```python
from build123d import *

# Parameters (mm, degrees)
BOSS_EXTRUDE1_DEPTH = 50.8
SKETCH2_W           = 28.5
SKETCH2_H           = 19.05
SKETCH2_H_2         = 62.95
SKETCH2_W_2         = 13.15
SKETCH2_H_3         = 42
CUT_EXTRUDE2_DEPTH  = 150
SKETCH8_R           = 9.625
CUT_EXTRUDE8_DEPTH  = 90.793902911
SKETCH11_R          = 9.625
SKETCH11_W          = 8.25
SKETCH11_H          = 8.25
BOSS_EXTRUDE4_DEPTH = 5.15
FILLET1_R           = 6
CUT_EXTRUDE10_START = -5.15
SKETCH14_R          = 1.5875
CUT_EXTRUDE10_DEPTH = 5.15
CUT_EXTRUDE16_REACH = 91.794
SKETCH21_R          = 3


with BuildPart() as part:
    # Sketch1 → Boss-Extrude1 (new body)
    with BuildSketch(Plane(origin=(0, 0, 0), x_dir=(0, 0, -1), z_dir=(1, 0, 0))):
        with BuildLine():
            Line((-52.5, 19.05), (52.5, 19.05))
            ThreePointArc((52.5, 19.05), (71.55, 0), (52.5, -19.05))
            Line((52.5, -19.05), (-52.5, -19.05))
            ThreePointArc((-52.5, -19.05), (-71.55, 0), (-52.5, 19.05))
        make_face()
    extrude(amount=BOSS_EXTRUDE1_DEPTH)

    # Sketch2 → Cut-Extrude2 (cut)
    with BuildSketch(Plane(origin=(0, 19.05, 0), x_dir=(1, 0, 0), z_dir=(0, 1, 0))):
        with Locations((25.4, 62.025)):
            Rectangle(SKETCH2_W, SKETCH2_H)
        with Locations((25.4, 21.025)):
            Rectangle(SKETCH2_W, SKETCH2_H_2)
        with Locations((44.225, -50.55)):
            Rectangle(SKETCH2_W_2, SKETCH2_H_3)
        with Locations((6.575, -50.55)):
            Rectangle(SKETCH2_W_2, SKETCH2_H_3)
    extrude(amount=-CUT_EXTRUDE2_DEPTH, mode=Mode.SUBTRACT)

    # Sketch8 → Cut-Extrude8 (cut, through all)
    with BuildSketch(Plane(origin=(50.8, 0, 0), x_dir=(0, 0, -1), z_dir=(1, 0, 0))):
        with Locations((-52.5, 0)):
            Circle(SKETCH8_R)
        with Locations((52.5, 0)):
            Circle(SKETCH8_R)
    extrude(amount=-CUT_EXTRUDE8_DEPTH, mode=Mode.SUBTRACT)

    # Sketch11 → Boss-Extrude4 (add)
    with BuildSketch(Plane(origin=(50.8, 0, 0), x_dir=(0, 0, -1), z_dir=(1, 0, 0))):
        with Locations((52.5, 0)):
            Circle(SKETCH11_R)
        with Locations((52.5, 0)):
            Rectangle(SKETCH11_W, SKETCH11_H, mode=Mode.SUBTRACT)
    extrude(amount=-BOSS_EXTRUDE4_DEPTH)

    # Fillet1
    fillet1_edges = [part.edges().sort_by_distance(p)[0] for p in [
        (50.8, 0, 29.55),
        (0, 0, 29.55),
    ]]
    fillet(fillet1_edges, radius=FILLET1_R)

    # Sketch14 → Cut-Extrude10 (cut)
    with BuildSketch(Plane(origin=(50.8, 0, 0), x_dir=(0, 0, -1), z_dir=(1, 0, 0)).offset(CUT_EXTRUDE10_START)):
        with Locations((49.497532015, 3.002467985)):
            Circle(SKETCH14_R)
        with Locations((55.502467985, 3.002467985)):
            Circle(SKETCH14_R)
        with Locations((55.502467985, -3.002467985)):
            Circle(SKETCH14_R)
        with Locations((49.497532015, -3.002467985)):
            Circle(SKETCH14_R)
    extrude(amount=CUT_EXTRUDE10_DEPTH, mode=Mode.SUBTRACT)

    # Sketch21 → Cut-Extrude16 (cut, up to next)
    with BuildSketch(Plane.ZY, mode=Mode.PRIVATE) as cut_extrude16_sk1:
        with Locations((-12.5, 13)):
            Circle(SKETCH21_R)
    cut_extrude16_tool1 = extrude(cut_extrude16_sk1.sketch, amount=-CUT_EXTRUDE16_REACH, mode=Mode.PRIVATE) & part.part
    # Sketch21 → Cut-Extrude16 (cut, up to next)
    with BuildSketch(Plane.ZY, mode=Mode.PRIVATE) as cut_extrude16_sk2:
        with Locations((-12.5, -13)):
            Circle(SKETCH21_R)
    cut_extrude16_tool2 = extrude(cut_extrude16_sk2.sketch, amount=-CUT_EXTRUDE16_REACH, mode=Mode.PRIVATE) & part.part
    add(cut_extrude16_tool1.solids().sort_by_distance((0, 13, -12.5))[0], mode=Mode.SUBTRACT)
    add(cut_extrude16_tool2.solids().sort_by_distance((0, -13, -12.5))[0], mode=Mode.SUBTRACT)


solid = part.part
```
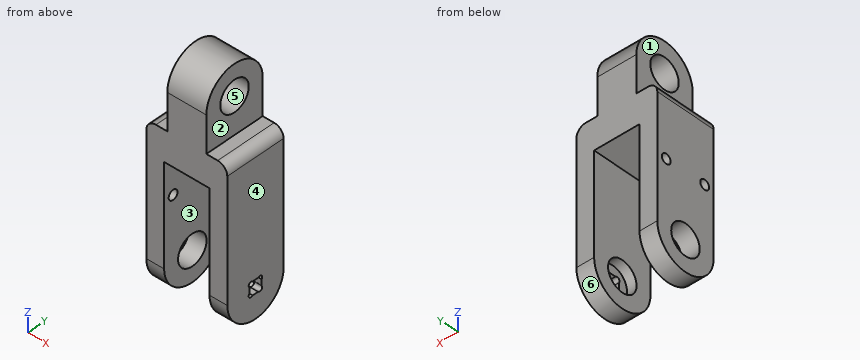
Geometry: final body of the model. Coordinates: model frame, mm. Face numbers are marked on the shaded views. A direction names the side the tool comes from. Give positions to 0.01 mm unless a question says otherwise; leave off trailing zeros. Loops run counter-clockwise (first coordinate to the right, second up) from the corner with the lowest first, then second, coordinate; pieces in that order, holes last. Notation, with made-up numbers: (-23, 57) -> (-10, 57) arc R11 cw to (-10, 68) -> close; hole circle Ø9 at (63, 30). An arc over 180 degrees is marked (long way). Use one line per item in the form item = value.
Item 1: Section query B-B on z = -31. Output: boundary loops of the cut face in (x, y), and give its area (3 significant figures).
A:
outline = (0, -19.05) -> (11.15, -19.05) -> (11.15, 19.05) -> (0, 19.05) -> close; (39.65, -19.05) -> (50.8, -19.05) -> (50.8, 19.05) -> (39.65, 19.05) -> close
area = 850 mm^2
Item 2: Draft query along Z for the marked faces 4, 5 and 6. Return one class per face: pulls with the +Z half, pulls with the -Z half, needs draft (parallel to the pull), parting line crosses it, or undercut.
A:
face_4 = needs draft
face_5 = undercut
face_6 = pulls with the -Z half
Item 3: Pin query (flat end, axial travel): P1, Ø5, axis at x = 18, y = 9, coming from the +Z side; P2, Ø2, axis at x = 41.5, y = -1.5, coming from the +Z side; P3, Ø6, axis at y = -3.5, z = -55, coming from the -X side. Return the tip coordinate at first contact, or that it passes through.
A:
P1 = 70.41
P2 = 29.55
P3 = 45.65
Item 4: Section query C-C on z = -12.5. Output: boundary loops of the cut face in (x, y), and give its area (3 significant figures).
A:
outline = (0, -19.05) -> (11.15, -19.05) -> (11.15, -16) -> (0, -16) -> close; (0, -10) -> (11.15, -10) -> (11.15, 10) -> (0, 10) -> close; (0, 16) -> (11.15, 16) -> (11.15, 19.05) -> (0, 19.05) -> close; (39.65, -19.05) -> (50.8, -19.05) -> (50.8, 19.05) -> (39.65, 19.05) -> close
area = 716 mm^2
Item 5: Line query: probe 1 along X at (y, z) = (2, -11); probe 2 along Y at (x, z) = (8, -12); probe 3 along Z at (x, y) = (39.5, 1.5). Output: solid intervals per line, ascending.
A:
probe_1 = 0 to 11.15, 39.65 to 50.8
probe_2 = -19.05 to -15.96, -10.04 to 10.04, 15.96 to 19.05
probe_3 = 10.45 to 29.55
Item 6: Section query A-A on y = 0. Give the number of separate pieces and of enclosed holes in the cut face, and give its area (3 significant figures).
A:
separate_pieces = 4
enclosed_holes = 0
area = 2,970 mm^2
Item 7: Access query for the marked faces 1, 2 and 3. Directions: +Z, -Z, +X, -X, +Y, -Y. A direction counts if a zero-diameter tool reaches every point of the face in a straight line with its end or side. Return the directions, or none.
A:
face_1 = +Z, -X, +Y, -Y
face_2 = +Z, +X, +Y, -Y
face_3 = -Z, +Y, -Y
Item 8: Section query D-D on y = 13. Output: boundary loops of the cut face in (x, z).
A:
outline = (0, -66.42) -> (11.15, -66.42) -> (11.15, -15.5) -> (0, -15.5) -> close; (0, -9.5) -> (11.15, -9.5) -> (11.15, 10.45) -> (39.65, 10.45) -> (39.65, -66.42) -> (50.8, -66.42) -> (50.8, 23.55) arc R6 ccw to (44.8, 29.55) -> (37.65, 29.55) -> (37.65, 66.42) -> (13.15, 66.42) -> (13.15, 29.55) -> (6, 29.55) arc R6 ccw to (0, 23.55) -> close
